The figure shows three views and two pictorial views of one solid part (mm, origin at its lowest corner). Answer the questions. Give positions to 0.01 mm unless a question says otherwise; leave off trailing zeros. Order: outer loops, then holes, each group sorted by start corner. A loop starts at its lowest first (then second) coordinate and runs counter-clockwise, first axis right, second up. Notation, with made-up numbers: M 74.25,71 L 114.25,71 A29 ccw 114.25,94 Z; hole C 6,83 d9. An arc over 180 degrees is marked long. Write item = value, one per line. Start each with the question number.
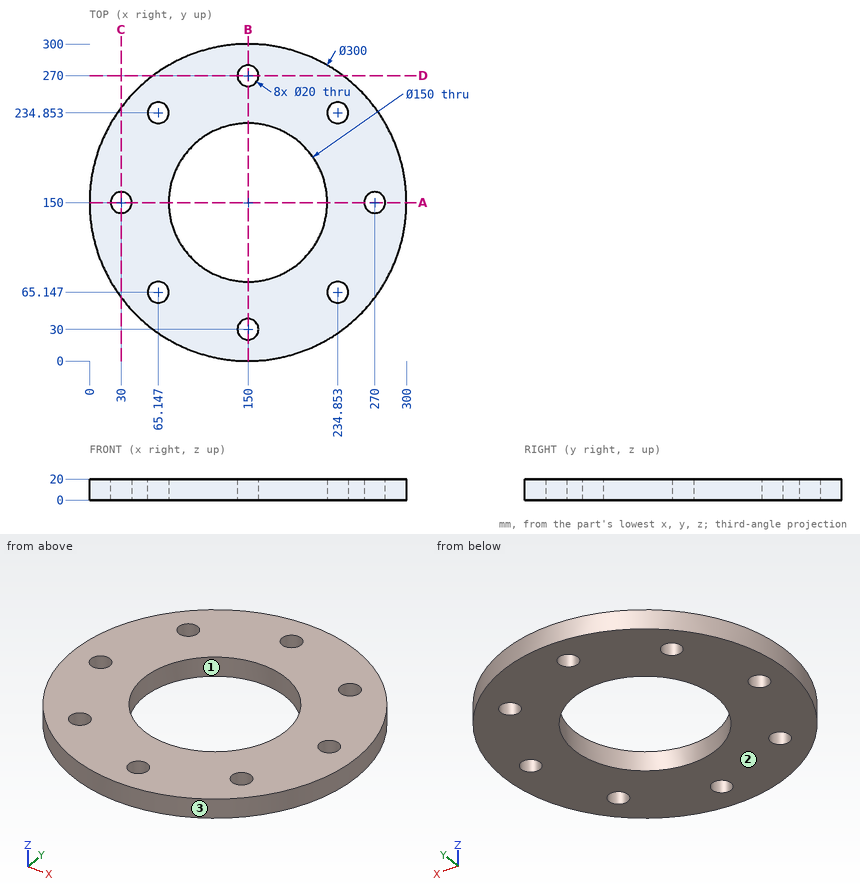
1) Find section A-A on y = 150. Determine the outline of the cut face in (x, z).
2) Find section C-C on x = 30. Determine the outline of the cut face in (y, z).
3) Each of these flat-tipped pins is pushed along its axis until it touches: P1, Ø2, axis at x = 84.5, z = 10, coming from the +Y side; P2, Ø10, axis at x = 89.5, z = 11, coming from the -Y side (1 decimal); P3, Ø4, axis at x = 70, z = 7, coming from the -Y side (1 decimal). Where does it stop, or does it pass through?
4) For a pull along X with two mould halves and no side action, classify the marked faces 1, 2 and 3 as pulls with the +X half, pulls with the -X half, needs draft (parallel to the pull), parting line crosses it, or undercut.
5) Find the intervals of material crossed by probe 1 along Y at (x, z) = (60, 16.5); probe 2 along Y at (x, z) = (65, 16); probe 3 along X at (y, z) = (261, 4.25), in increasing order. Write a range as [from, to].
Numbers:
q1.outline = M 0,0 L 20,0 L 20,20 L 0,20 Z; M 40,0 L 75,0 L 75,20 L 40,20 Z; M 225,0 L 260,0 L 260,20 L 225,20 Z; M 280,0 L 300,0 L 300,20 L 280,20 Z
q2.outline = M 60,0 L 140,0 L 140,20 L 60,20 Z; M 160,0 L 240,0 L 240,20 L 160,20 Z
q3.P1 = 285.42
q3.P2 = 10.6
q3.P3 = 21.9
q4.face_1 = undercut
q4.face_2 = needs draft
q4.face_3 = parting line crosses it
q5.probe_1 = [30, 56.57], [73.72, 226.28], [243.43, 270]
q5.probe_2 = [26.41, 55.15], [75.15, 224.85], [244.85, 273.59]
q5.probe_3 = [49.11, 145.64], [154.36, 250.89]
